Design review of the part built by this model. Coordinates are the model's own, in mm. Face numbers are marked on the shaded views. A direction names the side the tool comes from. Round coordinates to 2 decimals unless told otherwise and drop trailing zeros. Order: outer loops, then holes, each group sorted by start corner. A loop starts at its lowest first (then second) coordinate and runs counter-clockwise, first axis right, second up. Notation, with made-up numbers: (43, 0.25) - (70, 0.25) arc R11 cw to (70, 15.25) - close; hole circle Ø9 at (89.5, 81). An arc over 180 degrees is marked (long way). Write item = value, one per line.
from build123d import *

# Parameters (mm, degrees)
F0_R     = 17.5
F0_W     = 10
F0_H     = 30
F0_W_2   = 8
F0_H_2   = 15
F1_DEPTH = 25


with BuildPart() as f1:
    # F0 (on Top) → F1 (new body)
    with BuildSketch(Plane.XY):
        Polygon((68.0650311708, 32.2513162987), (-86.9349688292, 32.2513162987), (-86.9349688292, 7.2513162987), (-76.9349688292, 7.2513162987), (-69.0365880728, 7.2513162987), (-61.0365880728, 7.2513162987), (-52.6264092635, 7.2513162987), (-45.6264092635, 7.2513162987), (-38.6264092635, 7.2513162987), (68.0650311708, 7.2513162987), align=None)
        with BuildLine():
            ThreePointArc((68.0650311708, 7.2513162987), (135.7567732474, 19.7513162987), (68.0650311708, 32.2513162987))
            Line((68.0650311708, 32.2513162987), (68.0650311708, 7.2513162987))
        make_face()
        with Locations((100.7567732474, 19.7513162987)):
            Circle(F0_R, mode=Mode.SUBTRACT)
        with Locations((100.7567732474, 19.7513162987)):
            Circle(F0_R)
        with Locations((-81.9349688292, -7.7486837013)):
            Rectangle(F0_W, F0_H)
        with Locations((-65.0365880728, -0.2486837013)):
            Rectangle(F0_W_2, F0_H_2)
        Polygon((-45.6264092635, -7.7487440012), (-38.6264092635, 7.2513162987), (-45.6264092635, 7.2513162987), (-52.6264092635, 7.2513162987), align=None)
    extrude(amount=F1_DEPTH)


solid = f1.part
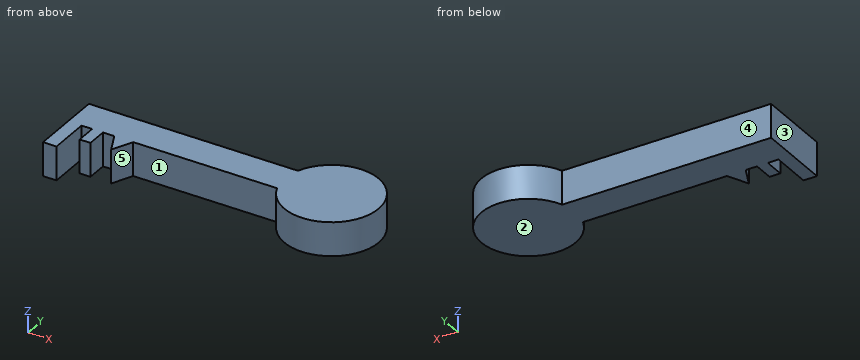
Item 1: Insertion check: P1, Ø6, axis at x = -16.5, z = 22, coming from the -Y side; P2, Ø7.5, axis at y = -2, z = 10.5, coming from the +X side; P3, Ø2.5, axis at x = -67, z = 9.5, coming from the -Y side. Each pin has a flat end and moves straight along its axis. Give the tip position at first contact, or say it passes through.
Data:
P1 = 7.25
P2 = 130.77
P3 = -7.75
Item 2: Take a section at A-A, the plane z = 2.75. State the section outline as (x, y) points, and give its area (3 significant figures).
Data:
outline = (-86.93, -22.75) - (-76.93, -22.75) - (-76.93, 7.25) - (-69.04, 7.25) - (-69.04, -7.75) - (-61.04, -7.75) - (-61.04, 7.25) - (-52.63, 7.25) - (-45.63, -7.75) - (-38.63, 7.25) - (68.07, 7.25) arc R35 ccw (long way) to (68.07, 32.25) - (-86.93, 32.25) - close
area = 8,210 mm2
Item 3: For the marked faces 1 and 2, list the 3-axis set-ups (+Z, -Z, +X, -X, +Y, -Y) from which the entire face can be reached by the end or side of a thin tool; tool diameter is ignored.
Data:
face_1 = +Z, -Z, -Y
face_2 = -Z, +X, -X, +Y, -Y
Item 4: Take a section at C-C, the plane x = -71. State the section outline as (y, z) points, and give its area (3 significant figures).
Data:
outline = (7.25, 0) - (32.25, 0) - (32.25, 25) - (7.25, 25) - close
area = 625 mm2
Item 5: The part is to be moulded in two halves that separate along X. For the marked faces 3, 4 and 5, say which applies: +X half, -X half, draft (parallel to the pull), parting line (faces both ways), or undercut.
Data:
face_3 = -X half
face_4 = draft
face_5 = undercut
Item 6: For line 1 along X through (y, z) = (-7, 10); line 2 along X through (y, z) = (-7.5, 17.25); line 3 along Y through (x, z) = (-42, 19.25), list the stretches that pass through material, from the lowest coordinate up. Write a range as [from, to].
Data:
line_1 = [-86.93, -76.93], [-69.04, -61.04], [-45.98, -45.28], [78.19, 123.33]
line_2 = [-86.93, -76.93], [-69.04, -61.04], [-45.74, -45.51], [78.79, 122.72]
line_3 = [0.02, 32.25]
Item 7: Take a section at B-B, the plane y = 46.5. State the section outline as (x, z) points, and give its area (3 significant figures).
Data:
outline = (78.18, 0) - (123.33, 0) - (123.33, 25) - (78.18, 25) - close
area = 1,130 mm2
